Can you work these out from the model? Positions are in its coordinate system, mm. A direction names the side the tool comes from. Round coordinates to 2 decimals unless told otherwise and drop trailing zeros. Order: outer loops, then holes, each group sorted by start corner. A loop starts at its lowest first (then second) coordinate and runs counter-clockwise, first axis right, second up. Notation, with made-up numbers: (54, -4.75) -> (84, -4.75) arc R23 ccw to (84, 26.25) -> close; hole circle Ø2 at (-18, 27.5). An arc over 180 degrees is marked (long way). One line per item, written item: value.
```python
from build123d import *

# Parameters (mm, degrees)
SKETCH_R        = 11.5
PAD_DEPTH       = 1.5
PAD001_DEPTH    = 5
FILLET_R        = 1
CHAMFER_1_SIZE2 = 0.45
CHAMFER_1_SIZE  = 1
CHAMFER_2_SIZE2 = 0.45
CHAMFER_2_SIZE  = 1


with BuildPart() as part:
    # Sketch → Pad (new body)
    with BuildSketch(Plane.XY):
        Circle(SKETCH_R)
    extrude(amount=PAD_DEPTH)

    # Sketch001 (on XY_Plane of Origin) → Pad001 (join)
    with BuildSketch(Plane.XY):
        with BuildLine():
            ThreePointArc((9.957052, 1.693258), (0.000108, 10.1), (-9.957015, 1.693471))
            ThreePointArc((-9.957015, 1.693471), (-9.547929, 1.116714), (-8.971172, 1.5258))
            ThreePointArc((8.971205, 1.525609), (9.7e-05, 9.1), (-8.971172, 1.5258))
            ThreePointArc((8.971205, 1.525609), (9.547953, 1.11651), (9.957052, 1.693258))
        make_face()
        with BuildLine():
            ThreePointArc((-9.957015, -1.693471), (0.000108, -10.1), (9.957052, -1.693258))
            ThreePointArc((9.957052, -1.693258), (9.547953, -1.11651), (8.971205, -1.525609))
            ThreePointArc((-8.971172, -1.5258), (9.7e-05, -9.1), (8.971205, -1.525609))
            ThreePointArc((-8.971172, -1.5258), (-9.547929, -1.116714), (-9.957015, -1.693471))
        make_face()
    extrude(amount=PAD001_DEPTH)

    # Fillet
    fillet_edges = [part.edges().sort_by_distance(p)[0] for p in [
        (-11.5, 0, 0),
    ]]
    fillet(fillet_edges, radius=FILLET_R)

    # Chamfer 1
    chamfer_1_edges = [part.edges().sort_by_distance(p)[0] for p in [
        (0.000108, 10.1, 5),
    ]]
    chamfer_1_side = part.faces().sort_by_distance((0.000108, 10.1, 3.25))[0]
    chamfer(chamfer_1_edges, length=CHAMFER_1_SIZE, length2=CHAMFER_1_SIZE2, reference=chamfer_1_side)

    # Chamfer 2
    chamfer_2_edges = [part.edges().sort_by_distance(p)[0] for p in [
        (0.000108, -10.1, 5),
    ]]
    chamfer_2_side = part.faces().sort_by_distance((0.000108, -10.1, 3.25))[0]
    chamfer(chamfer_2_edges, length=CHAMFER_2_SIZE, length2=CHAMFER_2_SIZE2, reference=chamfer_2_side)


solid = part.part
```
Q1. I want a section at B-B on y = 0. List the corners of the cut face in (x, z) for me.
Answers below:
outline: (-11.5, 1) arc R1 ccw to (-10.5, 0) -> (10.5, 0) arc R1 ccw to (11.5, 1) -> (11.5, 1.5) -> (-11.5, 1.5) -> close
Q2. I want a section at C-C on z = 0.55. List the corners of the cut face in (x, y) for me, plus the area to 3 significant figures.
Answers below:
outline: circle Ø22.79 at (0, 0)
area: 408 mm^2
Q3. Will these pins go through, and if not, where does the flat tip stop? pin 1 Ø1.5 at (x, y) = (7.5, 8.5) entering from -Z; pin 2 Ø1 at (x, z) = (3.5, 4) entering from -Y; pin 3 Ø1 at (x, z) = (5.5, 3) entering from -Y.
Answers below:
pin 1: z = 0
pin 2: y = -9.64
pin 3: y = -8.78
Q4. On a 3-axis mill with a long thin cutter (end or side, diameter ignored), from which of +Z, -Z, +X, -X, +Y, -Y can I reach the whole of each face in a straight line? I mean faces 4 (the face through (0.18, 9.1, 2.73)), 5 (the face through (-0.2, -10.1, 2.7)), 6 (the face through (0.2, 10.1, 2.7)). Say none if no direction works.
Answers below:
face 4: +Z
face 5: +Z, -Y
face 6: +Z, +Y
Q5. Please list where these lines run through material, in increasing order: line 1 along Y through (x, z) = (-0.25, 3.3); line 2 along Z through (x, y) = (-4, 6.5); line 3 along Y through (x, z) = (-3.25, 3.5).
Answers below:
line 1: -10.1 to -9.1, 9.1 to 10.1
line 2: 0 to 1.5
line 3: -9.56 to -8.5, 8.5 to 9.56
Q6. I want a section at A-A on z = 2.1. List the corners of the cut face in (x, y) for me.
Answers below:
outline: (-9.96, -1.69) arc R10.1 ccw to (9.96, -1.69) arc R0.5 ccw to (8.97, -1.53) arc R9.1 cw to (-8.97, -1.53) arc R0.5 ccw to start; (-9.96, 1.69) arc R0.5 ccw to (-8.97, 1.53) arc R9.1 cw to (8.97, 1.53) arc R0.5 ccw to (9.96, 1.69) arc R10.1 ccw to start
Q7. We'd pull the mould along Y, two halves only. Please class faces 1 (the face through (-1.5, 11.4, 1.2)), 2 (the face through (0, 0, 0)), 3 (the face through (-9.56, 1.12, 2.73)): released by +Y, released by -Y, zero draft, split by the parting line, or undercut.
Answers below:
face 1: split by the parting line
face 2: zero draft
face 3: undercut
